Check sheet for the modelled part. Datum: model origin and axes. Units: mm. A direction names the side the tool comes from. Round coordinates to 2 decimals unless told otherwise and drop trailing zeros. Order: outer loops, then holes, each group sorted by start corner. A loop starts at its lowest first (then second) coordinate and runs counter-clockwise, first axis right, second up.
from build123d import *

# Parameters (mm, degrees)
F0_R     = 2.15265
F0_R_2   = 1.7272
F1_DEPTH = 4.7625


# Not quite as in the source:
# - a feature names something its author has since deleted; it is built from what else it names


with BuildPart() as f1:
    # F0 (on Top) → F1 (new body)
    with BuildSketch(Plane.XY):
        with BuildLine():
            Line((22.3912242158, 0), (0, 0))
            Line((0, 0), (0, -10.5219006149))
            ThreePointArc((0, -10.5219006149), (0.4570421145, -15.9607009606), (5.9126458296, -15.8))
            Line((5.9126458296, -15.8), (28, -15.8))
            Line((28, -15.8), (28, -9.1773860778))
            Line((28, -9.1773860778), (43.1353352142, -18.980828941))
            ThreePointArc((43.1353352142, -18.980828941), (48.6239542062, -17.8073662506), (47.4504915157, -12.3187472586))
            Line((47.4504915157, -12.3187472586), (27.4575781507, 0.6310408412))
            ThreePointArc((27.4575781507, 0.6310408412), (24.809461921, 1.2383180364), (22.3912242158, 0))
        make_face()
        with Locations((3.1, -13)):
            Circle(F0_R, mode=Mode.SUBTRACT)
        with Locations((45.2929133649, -15.6497880998)):
            Circle(F0_R_2, mode=Mode.SUBTRACT)
        with Locations((31.96875, -7.0194754969)):
            Circle(F0_R_2, mode=Mode.SUBTRACT)
        with Locations((25.3, -2.7)):
            Circle(F0_R, mode=Mode.SUBTRACT)
    extrude(amount=F1_DEPTH)


solid = f1.part
1) Sectioned sample at B-B on y = -2.7. Record the cut outline in (x, z).
2) Sectioned sample at C-C on z = 0.8. Record the cut outline in (x, y), and give its area (3 significant figures).
3) Gauge pin test, flat ends, axial feed: pin 1 (2 mm diameter, centred on x = 11, z = 4.5, fed in from +Y); pin 2 (4 mm diameter, centred on x = 19, y = -15.5, fed in from -Z); pin 3 (1.4 mm diameter, centred on x = 17, z = 2, fed in from -Y); pin 4 (2 mm diameter, centred on y = -13, z = 2.5, fed in from +X). Record the tip position at first contact, or that the pin passes through.
4) Set-up check for faces 1 (the face through (17, -15.8, 2)), 2 (the face through (11, 0, 2)), 3 (the face through (2.63, -15.1, 2.35)): record each of +Z, -Z, +X, -X, +Y, -Y from which the full face is reachable in a straight line by a thin tool's end or side.
5) Scan lines: line 1 (X direction, y = -16.5, z = 2.4); line 2 (Y direction, x = 25.3, z = 2.35); line 3 (X direction, y = -15.25, z = 3.2). Record each from-to range of solid material in increasing order.
6) Sectioned sample at A-A on x = 3.1. Record the cut outline in (y, z).
7) Sectioned sample at D-D on x = 19.5. Record the cut outline in (y, z).
Values found:
1. outline: (0, 0) - (23.15, 0) - (23.15, 4.76) - (0, 4.76) - close; (27.45, 0) - (32.6, 0) - (32.6, 4.76) - (27.45, 4.76) - close
2. outline: (0, -10.52) arc R3.97 ccw to (5.91, -15.8) - (28, -15.8) - (28, -9.18) - (43.14, -18.98) arc R3.97 ccw to (47.45, -12.32) - (27.46, 0.63) arc R3.97 ccw to (22.39, 0) - (0, 0) - close; hole circle Ø4.31 at (3.1, -13); hole circle Ø4.31 at (25.3, -2.7); hole circle Ø3.45 at (31.97, -7.02); hole circle Ø3.45 at (45.29, -15.65)
2. area: 595 mm2
3. pin 1: stops at y = 0
3. pin 2: stops at z = 0
3. pin 3: stops at y = -15.8
3. pin 4: stops at x = 48.9
4. face 1: +Z, -Z, -Y
4. face 2: +Z, -Z, -X, +Y
4. face 3: +Z, -Z
5. line 1: x = 1.23 to 4.97, 39.31 to 43.79, 46.8 to 49.17
5. line 2: y = -15.8 to -4.85, -0.55 to 1.27
5. line 3: x = -0.17 to 28, 37.38 to 43.61, 46.97 to 49.24
6. outline: (-16.97, 0) - (-15.15, 0) - (-15.15, 4.76) - (-16.97, 4.76) - close; (-10.85, 0) - (0, 0) - (0, 4.76) - (-10.85, 4.76) - close
7. outline: (-15.8, 0) - (0, 0) - (0, 4.76) - (-15.8, 4.76) - close
